```python
from build123d import *

# Parameters (mm, degrees)
F0_W        = 54
F0_H        = 56
F1_DEPTH    = 3
F3_D        = 3.3
F3_DEPTH    = 4.55
F3_TIP      = 0.9914200214
F5_DEPTH    = 3.001
F7_D        = 3.3
F7_DEPTH    = 4.55
F7_TIP      = 0.9914200214
F8_T1_DEPTH = 29.9160411803
F8_T3_DEPTH = 30.4926194226
F8_T5_DEPTH = 30.4926194226
F8_T7_DEPTH = 29.9160411803
F9_R        = 3


# Not quite as in the source:
# - a fillet or chamfer that OpenCascade refuses, or shapes differently, is made with other operations: its cross-section is extruded or revolved along the edge and cut away or added


with BuildPart() as f1:
    # F0 (on Front) → F1 (new body)
    with BuildSketch(Plane.XZ):
        Rectangle(F0_W, F0_H)
    extrude(amount=F1_DEPTH)

    # F3
    with Locations(Plane.XZ.offset(3)):
        with Locations((-22.5, 22.5), (22.5, 22.5), (22.5, -22.5), (-22.5, -22.5)):
            Hole(F3_D / 2, depth=F3_DEPTH)
            with Locations((0, 0, -(F3_DEPTH + F3_TIP / 2))):  # 118° drill point
                Cone(0, F3_D / 2, F3_TIP, mode=Mode.SUBTRACT)

    # F4 (on face) → F5 (cut, through all)
    with BuildSketch(Plane.XZ.offset(3)):
        Polygon((-4.372583002, 0), (-27, 22.627416998), (-27, -22.627416998), align=None)
        Polygon((22.627416998, 28), (-22.627416998, 28), (0, 5.372583002), align=None)
        Polygon((27, -22.627416998), (27, 22.627416998), (4.372583002, 0), align=None)
        Polygon((0, -5.372583002), (-22.627416998, -28), (22.627416998, -28), align=None)
    extrude(amount=-F5_DEPTH, mode=Mode.SUBTRACT)

    # F7
    with Locations(Plane.XZ.offset(3)):
        with Locations((-9.5, 9.5), (9.5, 9.5), (9.5, -9.5), (-9.5, -9.5)):
            Hole(F7_D / 2, depth=F7_DEPTH)
            with Locations((0, 0, -(F7_DEPTH + F7_TIP / 2))):  # 118° drill point
                Cone(0, F7_D / 2, F7_TIP, mode=Mode.SUBTRACT)

    # F8: fillet of radius 5.5 on 4 edges, made by hand

    # F8_s2 → F8_t1 (cut)
    with BuildSketch(Plane.XZ.offset(-13.4580205902)):
        with BuildLine():
            ThreePointArc((-22.627416998, -28), (-25.7691213082, -26.0844427348), (-27, -22.6167917639))
            Line((-27, -22.6167917639), (-27, -28))
            Line((-27, -28), (-22.627416998, -28))
        make_face()
    extrude(amount=F8_T1_DEPTH, mode=Mode.SUBTRACT)

    # F8_s4 → F8_t3 (cut)
    with BuildSketch(Plane.XZ.offset(-13.7463097113)):
        with BuildLine():
            ThreePointArc((-27, 22.627416998), (-25.3452507259, 26.4338780795), (-21.5014761155, 28))
            Line((-21.5014761155, 28), (-27, 28))
            Line((-27, 28), (-27, 22.627416998))
        make_face()
    extrude(amount=F8_T3_DEPTH, mode=Mode.SUBTRACT)

    # F8_s6 → F8_t5 (cut)
    with BuildSketch(Plane.XZ.offset(-13.7463097113)):
        with BuildLine():
            ThreePointArc((27, -22.627416998), (25.3452507259, -26.4338780795), (21.5014761155, -28))
            Line((21.5014761155, -28), (27, -28))
            Line((27, -28), (27, -22.627416998))
        make_face()
    extrude(amount=F8_T5_DEPTH, mode=Mode.SUBTRACT)

    # F8_s8 → F8_t7 (cut)
    with BuildSketch(Plane.XZ.offset(-13.4580205902)):
        with BuildLine():
            ThreePointArc((22.627416998, 28), (25.7691213082, 26.0844427348), (27, 22.6167917639))
            Line((27, 22.6167917639), (27, 28))
            Line((27, 28), (22.627416998, 28))
        make_face()
    extrude(amount=F8_T7_DEPTH, mode=Mode.SUBTRACT)

    # F9
    f9_edges = [f1.edges().sort_by_distance(p)[0] for p in [
        (-27, -1.5, 22.627417),
        (-26.99999, -1.5, -22.627407),
        (27, -1.5, -22.627417),
        (26.99999, -1.5, 22.627407),
        (-22.627417, -1.5, -28),
        (22.530329, -1.5, -27.902912),
        (-22.530329, -1.5, 27.902912),
        (22.627417, -1.5, 28),
    ]]
    fillet(f9_edges, radius=F9_R)


solid = f1.part
```
Could you check a few things on this model? Use its own coordinates, in mm. A direction names the side the tool comes from. Round coordinates to 2 decimals unless told otherwise and drop trailing zeros. Order: outer loops, then holes, each group sorted by start corner. A loop starts at its lowest first (then second) coordinate and runs counter-clockwise, first axis right, second up. Notation, with made-up numbers: M 72,-12 L 116,-12 A16 ccw 116,17 Z; hole C 70.25,76.5 d7. An arc over 180 degrees is marked long. One line per question, with ' | ' between items. Start each with the question number.
(1) Suppose I cut it at A-A on z = 22.5. List the corners of the cut face in (x, y) for me.
(2) Please list where these lines run through material, in increasing order: line 1 along Z through (x, y) = (8, -1); line 2 along X through (y, z) = (-1.55, 8); line 3 along Z through (x, y) = (-9.5, -1.2).
(3) For faces 1 (the face through (26.009, -1.479, 25.766)), 2 (the face through (15.286, -1.521, 10.914)), which set-ups out of +Z, -Z, +X, -X, +Y, -Y let a thin tool reach every point of the face, with its end or its side?
(4) Suppose I cut it at C-C on y = -1.8. Count the separate pieces of the cut face and the enclosed holes in it, then the cut area to 3 significant figures.
(5) Suppose I cut it at D-D on z = -17. List the corners of the cut face in (x, y) for me, then the cut area to 3 significant figures.
(6) Suppose I cut it at B-B on x = -9.5. List the corners of the cut face in (y, z) for me.
(7) Thinking about a two-plate mould opening in Z: for faces 3 (the face through (-15.286, -1.521, -10.914)), 4 (the face through (23.716, -1.479, -21.385)), 5 (the face through (-10.69, -1.52, 16.06)), 6 (the face through (-10.42, -1.52, -15.79)), which applies, +Z half, -Z half, draft (parallel to the pull), parting line (faces both ways), or undercut?
Geometry results:
1) outline: M -26.53,-3 L -24.15,-3 L -24.15,0 L -26.53,0 Z; M -20.85,-3 L -17.13,-3 L -17.13,0 L -20.85,0 Z; M 17.13,-3 L 20.85,-3 L 20.85,0 L 17.13,0 Z; M 24.15,-3 L 26.55,-3 L 26.55,0 L 24.15,0 Z
2) line 1: -13.37 to -10.19, -8.81 to -3.63, 3.63 to 8.81, 10.19 to 13.37 | line 2: -12.37 to -10.19, -8.81 to -2.63, 2.63 to 8.81, 10.19 to 12.37 | line 3: -14.87 to -11.15, -7.85 to -5.13, 5.13 to 7.85, 11.15 to 14.87
3) face 1: +Z, +X, +Y, -Y | face 2: +X, +Y, -Y
4) separate pieces: 1 | enclosed holes: 8 | area: 877 mm²
5) outline: M -21.37,-3 L -11.63,-3 L -11.63,0 L -21.37,0 Z; M 11.63,-3 L 21.37,-3 L 21.37,0 L 11.63,0 Z | area: 58.5 mm²
6) outline: M -3,-14.87 L 0,-14.87 L 0,-11.15 L -3,-11.15 Z; M -3,-7.85 L 0,-7.85 L 0,-5.13 L -3,-5.13 Z; M -3,5.13 L 0,5.13 L 0,7.85 L -3,7.85 Z; M -3,11.15 L 0,11.15 L 0,14.87 L -3,14.87 Z
7) face 3: undercut | face 4: undercut | face 5: +Z half | face 6: -Z half
